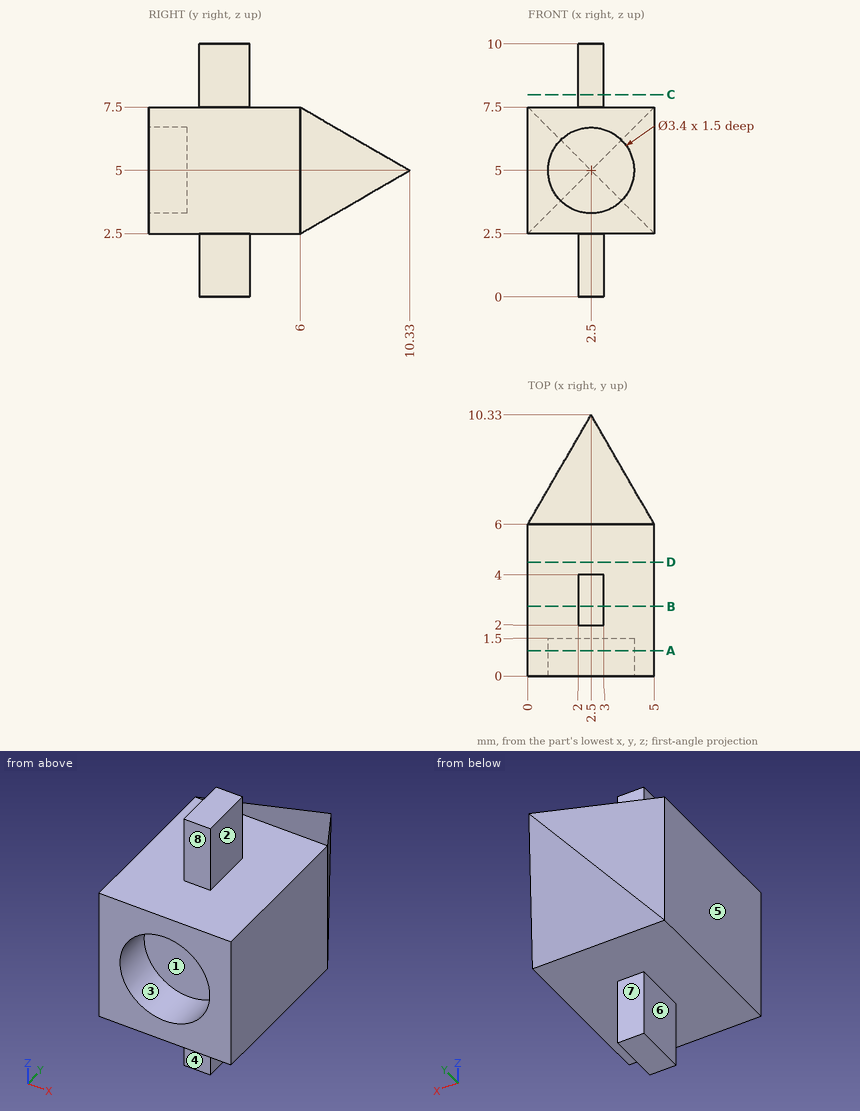
Geometry check sheet. Reference: drawing and pictorial views, mm from the part's lowest x, y, z. A direction names the side the tool comes from. Round coordinates to 2 decimals unless told otherwise and drop trailing zeros. Loops run counter-clockwise (first coordinate to the right, second up) from the corner with the lowest first, then second, coordinate; pieces in that order, holes last. Notation, with made-up numbers: (75.5, 17) - (112.5, 17) arc R25 cw to (112.5, 38) - close; hole circle Ø8 at (9, 29). An arc over 180 degrees is marked (long way). Use a Markdown table: item, result. Add a question column.
1. Release check for a two-part mould opening along X. For the marked faces 1, 2, 3 and 4 record: released by +X, released by -X, zero draft, split by the parting line, or undercut.
2. Section check A-A, the plane y = 1. Record the boundary of the cut face in (x, z), plus the area to 3 significant figures.
3. Access from +Z, -Z, +X, -X, +Y, -Y to the whole of each face (thin tool, end or side, straight path). Record for the marked faces 5, 6, 7 and 8.
4. Section check C-C, the plane z = 8. Record the boundary of the cut face in (x, y).
5. Gauge pin test, flat ends, axial feed: pin 1 (1.6 mm diameter, centred on y = 3, z = 0.5, fed in from -X); pin 2 (0.5 mm diameter, centred on x = 2.5, z = 1, fed in from -Y); pin 3 (0.6 mm diameter, centred on y = 2.5, z = 9, fed in from +X). Record the tip position at first contact, or that the pin passes through.
6. Section check D-D, the plane y = 4.5. Record the boundary of the cut face in (x, z).
7. Section check B-B, the plane y = 2.75. Record the boundary of the cut face in (x, z), plus the area to 3 significant figures.
8. Thickness scan on probe 1 along Z at (x, y) = (2.5, 1.2); probe 2 along X at (y, z) = (3.75, 9.25); probe 3 along X at (y, z) = (1, 4.75). Record the ranges inside material, lowest first. Write a range as [from, to].
Checks:
| question | item | result |
|---|---|---|
| 1 | face 1 | undercut |
| 1 | face 2 | released by +X |
| 1 | face 3 | undercut |
| 1 | face 4 | zero draft |
| 2 | outline | (0, 2.5) - (5, 2.5) - (5, 7.5) - (0, 7.5) - close; hole circle Ø3.4 at (2.5, 5) |
| 2 | area | 15.9 mm^2 |
| 3 | face 5 | +Z, -Z, -X, +Y, -Y |
| 3 | face 6 | -Z, -X, +Y, -Y |
| 3 | face 7 | -Z, +X, -X, +Y |
| 3 | face 8 | +Z, +X, -X, -Y |
| 4 | outline | (2, 2) - (3, 2) - (3, 4) - (2, 4) - close |
| 5 | pin 1 | stops at x = 2 |
| 5 | pin 2 | stops at y = 2 |
| 5 | pin 3 | stops at x = 3 |
| 6 | outline | (0, 2.5) - (5, 2.5) - (5, 7.5) - (0, 7.5) - close |
| 7 | outline | (0, 2.5) - (2, 2.5) - (2, 0) - (3, 0) - (3, 2.5) - (5, 2.5) - (5, 7.5) - (3, 7.5) - (3, 10) - (2, 10) - (2, 7.5) - (0, 7.5) - close |
| 7 | area | 30.0 mm^2 |
| 8 | probe 1 | z = [2.5, 3.3], [6.7, 7.5] |
| 8 | probe 2 | x = [2, 3] |
| 8 | probe 3 | x = [0, 0.82], [4.18, 5] |
